```python
from build123d import *

# Parameters (mm, degrees)
F0_R     = 50
F1_DEPTH = 43
F2_R     = 29.25
F3_DEPTH = 35.5
F4_R     = 15
F5_R     = 9.5
F6_DEPTH = 8


with BuildPart() as f1:
    # F0 (on Top) → F1 (new body)
    with BuildSketch(Plane.XY):
        Circle(F0_R)
    extrude(amount=F1_DEPTH)

    # F2 (on face) → F3 (cut)
    with BuildSketch(Plane.XY.offset(43)):
        Circle(F2_R)
    extrude(amount=-F3_DEPTH, mode=Mode.SUBTRACT)

    # F4
    f4_edges = [f1.edges().sort_by_distance(p)[0] for p in [
        (-50, 0, 0),
    ]]
    fillet(f4_edges, radius=F4_R)

    # F5 (on face) → F6 (cut)
    with BuildSketch(Plane(origin=(0, 0, 0), x_dir=(1, 0, 0), z_dir=(0, 0, -1))):
        Circle(F5_R)
    extrude(amount=-F6_DEPTH, mode=Mode.SUBTRACT)


solid = f1.part
```
CAD build for the part. Positions are in the model's coordinates, mm. A direction names the side the tool comes from. Give positions to 0.01 mm unless a question says otherwise; leave off trailing zeros. Order: outer loops, then holes, each group sorted by start corner. A loop starts at its lowest first (then second) coordinate and runs counter-clockwise, first axis right, second up.
(1) Flat gauge pins, fed straight in: pin 1 (3 mm diameter, centred on y = -18, z = 28, fed in from -X); pin 2 (10 mm diameter, centred on x = 3.5, z = 8.5, fed in from -Y); pin 3 (1.5 mm diameter, centred on x = -8.5, z = 27.5, fed in from -Y); pin 4 (17 mm diameter, centred on x = 0, y = 0, fed in from +Z). Where does each tip first touch, or does it go through?
(2) Tool access for faces 1 (the flat face through (22, -22, 43)), 2 (the cylindrical face through (-6.341, -28.554, 25.498)): list every direction of +Z, -Z, +X, -X, +Y, -Y with a clear straight run to the whole face (end or side of a thin tool).
(3) Saw through at A-A, the plane x = 0. Give the cut face in (y, z), then the cut area to 3 significant figures.
(4) Mould opens along Y. For faces 3 (the cylindrical face through (4.38, 8.43, 3.7)), 4 (the flat face through (7, -7, 0)), 5 (the cylindrical face through (47.69, 15.02, 28.8)) say: released by +Y, released by -Y, zero draft, split by the parting line, or undercut.
(5) Saw through at C-C, the plane z = 27. Give the cut face in (x, y), then the cut area to 3 significant figures.
(6) Drill centre lines: L1, parallel to Y at x = 0, z = 36; L2, parallel to Z at x = 4.5, y = 35.5; L3, parallel to Z at x = -21, y = -9. Where is each one in solid material? Low to high.
(7) Saw through at D-D, the plane z = 13.5. Give the cut face in (x, y), then the cut area to 3 significant figures.
Results found:
1. pin 1: stops at x = -47.2
1. pin 2: stops at y = -49.86
1. pin 3: stops at y = -49.4
1. pin 4: passes through
2. face 1: +Z, +X, -X, +Y, -Y
2. face 2: +Z
3. outline: (-50, 15) arc R15 ccw to (-35, 0) - (-9.5, 0) - (-9.5, 7.5) - (-29.25, 7.5) - (-29.25, 43) - (-50, 43) - close; (9.5, 0) - (35, 0) arc R15 ccw to (50, 15) - (50, 43) - (29.25, 43) - (29.25, 7.5) - (9.5, 7.5) - close
3. area: 1,980 mm2
4. face 3: undercut
4. face 4: zero draft
4. face 5: split by the parting line
5. outline: circle Ø100 at (0, 0); hole circle Ø58.5 at (0, 0)
5. area: 5,170 mm2
6. L1: y = -50 to -29.25, 29.25 to 50
6. L2: z = 0.02 to 43
6. L3: z = 0 to 7.5
7. outline: circle Ø99.85 at (0, 0); hole circle Ø58.5 at (0, 0)
7. area: 5,140 mm2
